Autodesk Inventor part; units mm, degrees
ref_plane "Work Plane1" through (0, 0, 0) normal (0, 0, 1) x (1, 0, 0)
ref_plane "Work Plane2" through (0, 0, 244.475) normal (0, 0, 1) x (1, 0, 0)
ref_plane "YZ Plane" through (0, 0, 0) normal (1, 0, 0) x (0, 1, 0)
ref_plane "Work Plane1" through (0, 0, 0) normal (0, 0, 1) x (1, 0, 0)
sketch "Sketch1" plane through (0, 0, 0) normal (0, 0, 1) x (1, 0, 0)
  arc A0 (-113.2188, 0) -> (-109.7581, 3.4607) centre (-113.2188, 3.4607) ccw
  line L0 (-109.7581, 17.1767) -> (-109.7581, 3.4607)
  arc A1 (-109.7581, 17.1767) -> (-114.8063, 22.225) centre (-114.8063, 17.1767) ccw
  line L1 (-115.8223, 22.225) -> (-114.8063, 22.225)
  arc A2 (-115.8223, 22.225) -> (-119.2831, 18.7642) centre (-115.8223, 18.7642) ccw
  line L2 (-119.2831, 16.4211) -> (-119.2831, 18.7642)
  arc A3 (-119.2831, 16.4211) -> (-116.6161, 16.4211) centre (-117.9496, 16.4211) ccw
  line L3 (-116.6161, 18.7642) -> (-116.6161, 16.4211)
  arc A4 (-115.8223, 19.558) -> (-116.6161, 18.7642) centre (-115.8223, 18.7642) ccw
  line L4 (-114.8063, 19.558) -> (-115.8223, 19.558)
  arc A5 (-112.4251, 17.1767) -> (-114.8063, 19.558) centre (-114.8063, 17.1767) ccw
  line L5 (-112.4251, 3.4607) -> (-112.4251, 17.1767)
  arc A6 (-113.2188, 2.667) -> (-112.4251, 3.4607) centre (-113.2188, 3.4607) ccw
  line L6 (-147.5723, 2.667) -> (-113.2188, 2.667)
  arc A7 (-148.3661, 3.4607) -> (-147.5723, 2.667) centre (-147.5723, 3.4607) ccw
  line L7 (-148.3661, 17.1767) -> (-148.3661, 3.4607)
  arc A8 (-145.9848, 19.558) -> (-148.3661, 17.1767) centre (-145.9848, 17.1767) ccw
  line L8 (-144.9688, 19.558) -> (-145.9848, 19.558)
  arc A9 (-144.1751, 18.7642) -> (-144.9688, 19.558) centre (-144.9688, 18.7642) ccw
  line L9 (-144.1751, 16.4211) -> (-144.1751, 18.7642)
  arc A10 (-144.1751, 16.4211) -> (-141.5081, 16.4211) centre (-142.8416, 16.4211) ccw
  line L10 (-141.5081, 18.7642) -> (-141.5081, 16.4211)
  arc A11 (-141.5081, 18.7642) -> (-144.9688, 22.225) centre (-144.9688, 18.7642) ccw
  line L11 (-145.9848, 22.225) -> (-144.9688, 22.225)
  arc A12 (-145.9848, 22.225) -> (-151.0331, 17.1767) centre (-145.9848, 17.1767) ccw
  line L12 (-151.0331, 3.4607) -> (-151.0331, 17.1767)
  arc A13 (-151.0331, 3.4607) -> (-147.5723, 0) centre (-147.5723, 3.4607) ccw
  line L13 (-113.2188, 0) -> (-147.5723, 0)
  point P0 (0, 0)
extrude "Extrusion1" add sketch "Sketch1" along normal blind 488.95
ref_plane "Work Plane2" through (0, 0, 244.475) normal (0, 0, 1) x (1, 0, 0)
properties part number "Horizontal-Unistrut-Tower-Connector-19-25"
Source: CAD feature listing. Evaluate the final solid. Frame: model axes, mm. A direction names the side the tool comes from. Give positions to 0.01 mm unless a question says otherwise; leave off trailing zeros. Order: outer loops, then holes, each group sorted by start corner. A loop starts at its lowest first (then second) coordinate and runs counter-clockwise, first axis right, second up. Notation, with made-up numbers: (21, 29.5) -> (51, 29.5) arc R19 cw to (51, 40.5) -> close; hole circle Ø2 at (7, 45.5). An arc over 180 degrees is marked (long way). Use a Markdown table: item, result.
Q1. Section C-C (x = -131.5). Return the cut outline in (y, z).
A:
| item | result |
|---|---|
| outline | (0, 0) -> (2.67, 0) -> (2.67, 488.95) -> (0, 488.95) -> close |
Q2. Material intervals for line 1 (X direction, y = 17.75, z = 309); line 2 (X direction, y = 17.25, z = 237.5); line 3 (X direction, y = 3.75, z = 419), sorted ascending. Write a range as [from, to].
A:
| item | result |
|---|---|
| line 1 | [-151, -148.3], [-144.18, -141.51], [-119.28, -116.62], [-112.5, -109.79] |
| line 2 | [-151.03, -148.36], [-144.18, -141.51], [-119.28, -116.62], [-112.43, -109.76] |
| line 3 | [-151.03, -148.37], [-112.43, -109.76] |
Q3. First-contact query: P1, Ø10, axis at x = -124.5, z = 232.5, coming from the +Y side; P2, Ø1.2, axis at y = 18, z = 345.5, coming from the +X side. Flat tips, straight axial feed; report the tip coordinate or a pass-through.
A:
| item | result |
|---|---|
| P1 | y = 2.67 |
| P2 | x = -109.76 |
Q4. Access query for faces 4 (the face through (-130, 2, 488.95)), 5 (the face through (-131, 2.667, 241)). Directions: +Z, -Z, +X, -X, +Y, -Y. A direction counts if a zero-diameter tool reaches every point of the face in a straight line with its end or side. Return the directions, or none.
A:
| item | result |
|---|---|
| face 4 | +Z, +X, -X, +Y, -Y |
| face 5 | +Z, -Z |
Q5. Section A-A (y = 9). Return the cut outline in (x, z).
A:
| item | result |
|---|---|
| outline | (-151.03, 0) -> (-148.37, 0) -> (-148.37, 488.95) -> (-151.03, 488.95) -> close; (-112.43, 0) -> (-109.76, 0) -> (-109.76, 488.95) -> (-112.43, 488.95) -> close |
Q6. Section B-B (z = 432.5). Return the cut outline in (x, y) (1 decimal), and give its area (3 significant figures).
A:
| item | result |
|---|---|
| outline | (-151, 3.5) arc R3.5 ccw to (-147.6, 0) -> (-113.2, 0) arc R3.5 ccw to (-109.8, 3.5) -> (-109.8, 17.2) arc R5 ccw to (-114.8, 22.2) -> (-115.8, 22.2) arc R3.5 ccw to (-119.3, 18.8) -> (-119.3, 16.4) arc R1.3 ccw to (-116.6, 16.4) -> (-116.6, 18.8) arc R0.8 cw to (-115.8, 19.6) -> (-114.8, 19.6) arc R2.4 cw to (-112.4, 17.2) -> (-112.4, 3.5) arc R0.8 cw to (-113.2, 2.7) -> (-147.6, 2.7) arc R0.8 cw to (-148.4, 3.5) -> (-148.4, 17.2) arc R2.4 cw to (-146, 19.6) -> (-145, 19.6) arc R0.8 cw to (-144.2, 18.8) -> (-144.2, 16.4) arc R1.3 ccw to (-141.5, 16.4) -> (-141.5, 18.8) arc R3.5 ccw to (-145, 22.2) -> (-146, 22.2) arc R5 ccw to (-151, 17.2) -> close |
| area | 255 mm^2 |
Q7. Pull-direction query (Y, two-part tool) for faces 1 (the face through (-130, 0, 241)), 2 (the face through (-109.758, 10, 241)), 3 (the face through (-112.425, 10, 241)); classes: +Y half, -Y half, draft (parallel to the pull), parting line (faces both ways), or undercut.
A:
| item | result |
|---|---|
| face 1 | -Y half |
| face 2 | draft |
| face 3 | undercut |
